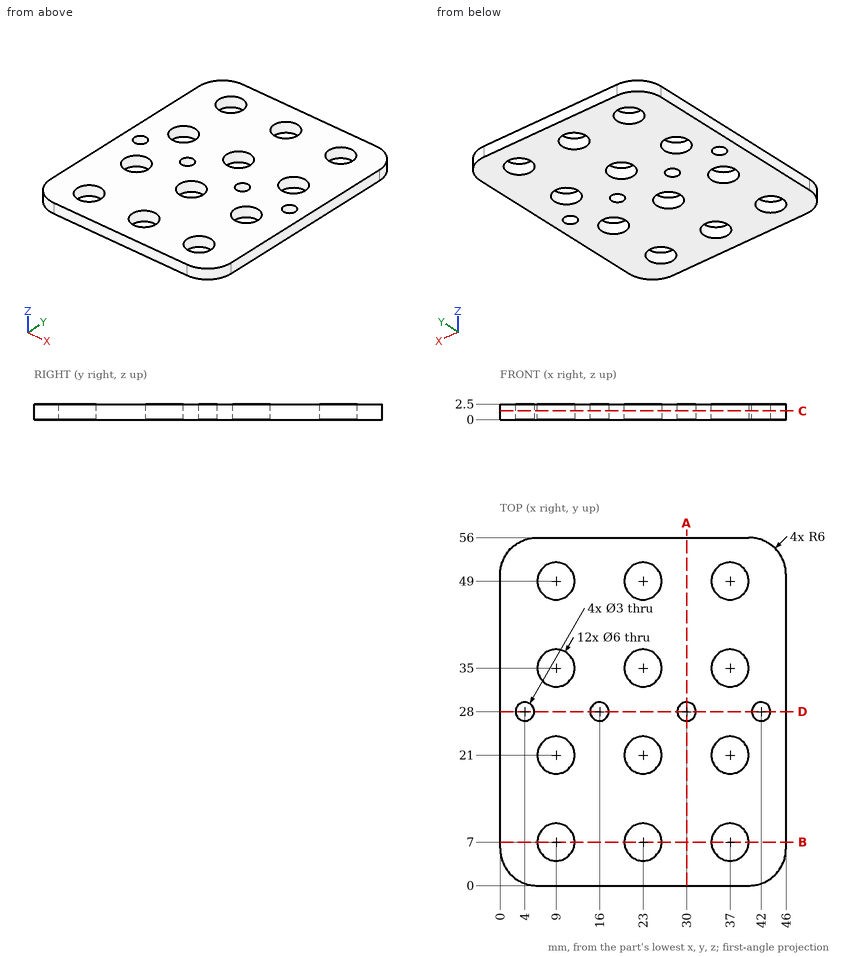
Geometry: see drawing. Coordinates: mm, zero at the bounding-box minimum. Give positions to 0.01 mm unless a question says otherwise; leave off trailing zeros. Order: outer loops, then holes, each group sorted by start corner. A loop starts at its lowest first (then second) coordinate and runs counter-clockwise, first axis right, second up. Notation, with made-up numbers: (-35, 82) - (5, 82) arc R15 cw to (5, 107) - close; hole circle Ø11 at (-9, 38.5). An arc over 180 degrees is marked (long way). Write each question's results on one line, items separated by ' | '.
Item 1: Section A-A (x = 30). Return loops of the section in (y, z), and give its area (4 significant figures).
A:
outline: (0, 0) - (26.5, 0) - (26.5, 2.5) - (0, 2.5) - close; (29.5, 0) - (56, 0) - (56, 2.5) - (29.5, 2.5) - close | area: 132.5 mm^2
Item 2: Material intervals for line 1 along Y through (x, z) = (37, 0.9); line 2 along Y through (x, z) = (36, 2.4); line 3 along X through (y, z) = (20, 0.45), sorted ascending.
A:
line 1: y = 0 to 4, 10 to 18, 24 to 32, 38 to 46, 52 to 56 | line 2: y = 0 to 4.17, 9.83 to 18.17, 23.83 to 32.17, 37.83 to 46.17, 51.83 to 56 | line 3: x = 0 to 6.17, 11.83 to 20.17, 25.83 to 34.17, 39.83 to 46
Item 3: Contact query for a flat-ended pin moving along its axis: pin 1 Ø1.5 at (y, z) = (42.5, 1) entering from -X. Output: stop coordinate, or through.
A:
pin 1: stops at x = 0
Item 4: Section D-D (y = 28). Return loops of the section in (x, z).
A:
outline: (0, 0) - (2.5, 0) - (2.5, 2.5) - (0, 2.5) - close; (5.5, 0) - (14.5, 0) - (14.5, 2.5) - (5.5, 2.5) - close; (17.5, 0) - (28.5, 0) - (28.5, 2.5) - (17.5, 2.5) - close; (31.5, 0) - (40.5, 0) - (40.5, 2.5) - (31.5, 2.5) - close; (43.5, 0) - (46, 0) - (46, 2.5) - (43.5, 2.5) - close
Item 5: Section B-B (y = 7). Return loops of the section in (x, z).
A:
outline: (0, 0) - (6, 0) - (6, 2.5) - (0, 2.5) - close; (12, 0) - (20, 0) - (20, 2.5) - (12, 2.5) - close; (26, 0) - (34, 0) - (34, 2.5) - (26, 2.5) - close; (40, 0) - (46, 0) - (46, 2.5) - (40, 2.5) - close
Item 6: Section C-C (z = 1.4). Give the number of separate pieces and of enclosed holes in the cut face, and give its area (3 significant figures).
A:
separate pieces: 1 | enclosed holes: 16 | area: 2,180 mm^2
